Verification items for the finished model (mm, model axes). Give positions to 0.01 mm unless a question says otherwise; leave off trailing zeros. Loops run counter-clockwise (first coordinate to the right, second up) from the corner with the lowest first, then second, coordinate; pieces in that order, holes last. Notation, with made-up numbers: M -19.75,57 L 9.25,57 A14 cw 9.25,63 Z; hole C 16.25,37 d11. An arc over 180 degrees is marked long. Use a Markdown table: item, result.
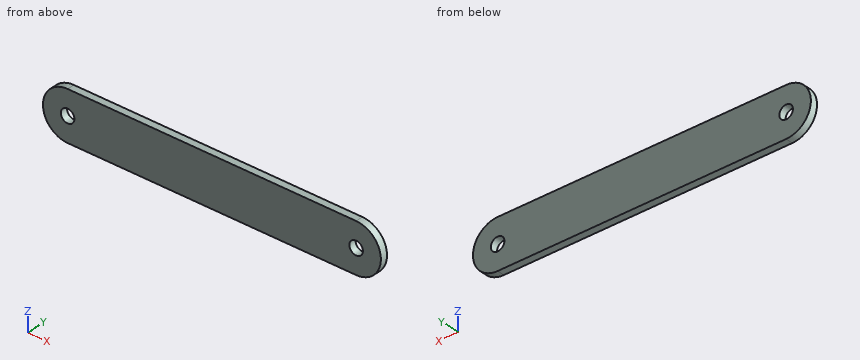
from build123d import *

# Parameters (mm, degrees)
EXTRUDE_1_DEPTH     = 3
SKETCH_2_R          = 5.5
CUT_EXTRUDE_1_DEPTH = 9


with BuildPart() as part:
    # 草图1 → 凸台-拉伸1 (new, symmetric)
    with BuildSketch(Plane(origin=(0, 0, 0), x_dir=(1, 0, 0), z_dir=(0, 1, 0))):
        with BuildLine():
            Line((116.85, -20), (-116.85, -20))
            ThreePointArc((-116.85, -20), (-136.85, 0), (-116.85, 20))
            Line((-116.85, 20), (116.85, 20))
            ThreePointArc((116.85, 20), (136.85, 0), (116.85, -20))
        make_face()
    extrude(amount=EXTRUDE_1_DEPTH, both=True)

    # 草图2 → 切除-拉伸1 (cut)
    with BuildSketch(Plane(origin=(0, 3, 0), x_dir=(1, 0, 0), z_dir=(0, 1, 0))):
        with Locations(Location((-116.85, 0, 0), (0, 0, 270))):
            Circle(SKETCH_2_R)
        with Locations(Location((116.85, 0, 0), (0, 0, 270))):
            Circle(SKETCH_2_R)
    extrude(amount=-CUT_EXTRUDE_1_DEPTH, mode=Mode.SUBTRACT)


solid = part.part
(1) Gauge pin test, flat ends, axial feed: P1, Ø1.5, axis at y = -0.5, z = -14.5, coming from the -X side; P2, Ø12.5, axis at x = 116.85, z = 0, coming from the +Y side; P3, Ø1.5, axis at y = 2, z = -11, coming from the -X side. Record the tip position at first contact, or that the pin passes through.
Results below:
| item | result |
|---|---|
| P1 | x = -131.37 |
| P2 | y = 3 |
| P3 | x = -134.02 |
(2) Material ranges on line 1 (X direction, y = 0.7, z = 0); line 2 (X direction, y = 2.2, z = -4); line 3 (Z direction, x = -117, y = -0.65), recorded low to high.
Results below:
| item | result |
|---|---|
| line 1 | -136.85 to -122.35, -111.35 to 111.35, 122.35 to 136.85 |
| line 2 | -136.45 to -120.62, -113.08 to 113.08, 120.62 to 136.45 |
| line 3 | -20 to -5.5, 5.5 to 20 |
(3) Cross-section at A-A on z = 0. Record the cut outline in (x, y).
Results below:
| item | result |
|---|---|
| outline | M -136.85,-3 L -122.35,-3 L -122.35,3 L -136.85,3 Z; M -111.35,-3 L 111.35,-3 L 111.35,3 L -111.35,3 Z; M 122.35,-3 L 136.85,-3 L 136.85,3 L 122.35,3 Z |
(4) Cross-section at C-C on z = 13.5. Record the cut outline in (x, y).
Results below:
| item | result |
|---|---|
| outline | M -131.61,-3 L 131.61,-3 L 131.61,3 L -131.61,3 Z |
(5) Cross-section at B-B on y = -1.35. Record the cut outline in (x, z).
Results below:
| item | result |
|---|---|
| outline | M -116.85,-20 L 116.85,-20 A20 ccw 116.85,20 L -116.85,20 A20 ccw Z; hole C -116.85,0 d11; hole C 116.85,0 d11 |
